```python
from build123d import *

# Parameters (mm, degrees)
SKETCH1_W           = 650
SKETCH1_H           = 250
SKETCH1_R           = 12.5
BOSS_EXTRUDE1_DEPTH = 119
SKETCH2_R           = 75
CUT_EXTRUDE1_DEPTH  = 267
FILLET1_R           = 50


with BuildPart() as part:
    # Sketch1 → Boss-Extrude1 (new body, symmetric)
    with BuildSketch(Plane(origin=(0, 0, 0), x_dir=(1, 0, 0), z_dir=(0, 1, 0))):
        Rectangle(SKETCH1_W, SKETCH1_H)
        with Locations((-250, -75)):
            Circle(SKETCH1_R, mode=Mode.SUBTRACT)
        with Locations((250, -75)):
            Circle(SKETCH1_R, mode=Mode.SUBTRACT)
        with Locations((250, 50)):
            Circle(SKETCH1_R, mode=Mode.SUBTRACT)
        with Locations((-250, 50)):
            Circle(SKETCH1_R, mode=Mode.SUBTRACT)
    extrude(amount=BOSS_EXTRUDE1_DEPTH, both=True)

    # Sketch2 → Cut-Extrude1 (cut)
    with BuildSketch(Plane.XY.offset(125)):
        with BuildLine():
            Line((-35.156791662, 87), (-325, 87))
            Line((-325, 87), (-325, -119))
            Line((-325, -119), (-5.04e-07, -119))
            ThreePointArc((-5.04e-07, -119), (-104.489233938, -30.832554252), (-35.156791662, 87))
        make_face()
        with BuildLine():
            Line((325, -119), (325, 87))
            Line((325, 87), (35.156791662, 87))
            ThreePointArc((35.156791662, 87), (104.489233853, -30.832554748), (-5.04e-07, -119))
            Line((-5.04e-07, -119), (325, -119))
        make_face()
        with Locations((0, -13)):
            Circle(SKETCH2_R)
    extrude(amount=-CUT_EXTRUDE1_DEPTH, mode=Mode.SUBTRACT)

    # Fillet1
    fillet1_edges = [part.edges().sort_by_distance(p)[0] for p in [
        (-35.156791662, 87, 0),
        (35.156791662, 87, 0),
    ]]
    fillet(fillet1_edges, radius=FILLET1_R)


solid = part.part
```
For this review, take the finished solid that the model builds, in its own axes (mm). A direction names the side the tool comes from. Give positions to 0.01 mm unless a question says otherwise; leave off trailing zeros. Write each loop counter-clockwise with the first axis right and the second up, starting at its lowest first coordinate (ties: lowest second). Pieces come first, ordered by that corner, then holes.
Item 1: Take a section at B-B (y = -13). Give the boundary of the cut face in (x, z), and give its area (3 significant figures).
Item 2: Insertion check: P1, Ø5, axis at x = 55.5, z = -18.5, coming from the -Y side; P2, Ø2, axis at y = -35.5, z = -71, coming from the +X side; P3, Ø1, axis at x = 76.5, z = 5.5, coming from the -Y side. Each pin has a flat end and moves straight along its axis. Give the tip position at first contact, or say it passes through.
Item 3: Machinability: for faces 1 (the face through (261.923, 102.776, -53.755)), 2 (the face through (238, 87, 2)), which of the approach directions +Z, -Z, +X, -X, +Y, -Y give a long, thin tool a straight path to every point of the face, cutting with its end or side? Answer none if there is none.
Item 4: The part is to be moulded in two halves that separate along Y. For faces 3 (the face through (-235, 87, 2)), 4 (the face through (-5, 119, -2)), 5 (the face through (-325, 103, 2)), 6 (the face through (107.53, 66.68, -1.75)), say which applies: +Y half, -Y half, draft (parallel to the pull), parting line (faces both ways), or undercut.
Item 5: Take a section at A-A (x = -250). Give the boundary of the cut face in (y, z), and give its area (3 significant figures).
Item 6: Wall thickness on probe 1 along X at (y, z) = (96, 75); probe 2 along Z at (x, y) = (250, 107); probe 3 along Y at (x, z) = (0, -1): over which ranges is each line inside the solid? List them lowest first.
Item 7: Take a section at C-C (z = 75). Give the boundary of the cut face in (x, y).
Item 8: Take a section at D-D (x = -65). Give the boundary of the cut face in (y, z), and give its area (3 significant figures).
Established:
1. outline: (-106, -125) - (-75, -125) - (-75, 125) - (-106, 125) - close; (75, -125) - (106, -125) - (106, 125) - (75, 125) - close
1. area: 15,500 mm2
2. P1: stops at y = -104.8
2. P2: stops at x = 103.8
2. P3: stops at y = -86.89
3. face 1: +Y, -Y
3. face 2: +Z, -Z, +X, -Y
4. face 3: -Y half
4. face 4: +Y half
4. face 5: draft
4. face 6: undercut
5. outline: (87, -125) - (119, -125) - (119, -62.5) - (87, -62.5) - close; (87, -37.5) - (119, -37.5) - (119, 62.5) - (87, 62.5) - close; (87, 87.5) - (119, 87.5) - (119, 125) - (87, 125) - close
5. area: 6,400 mm2
6. probe 1: x = -325 to -262.5, -237.5 to 237.5, 262.5 to 325
6. probe 2: z = -125 to -62.5, -37.5 to 62.5, 87.5 to 125
6. probe 3: y = -119 to -88, 62 to 119
7. outline: (-325, 87) - (-262.5, 87) - (-262.5, 119) - (-325, 119) - close; (-237.5, 87) - (-147.77, 87) arc R50 cw to (-100.41, 20.97) arc R106 ccw (long way) to (100.41, 20.97) arc R50 cw to (147.77, 87) - (237.5, 87) - (237.5, 119) - (-237.5, 119) - close; (262.5, 87) - (325, 87) - (325, 119) - (262.5, 119) - close; hole circle Ø150 at (0, -13)
8. outline: (-96.73, -125) - (-50.42, -125) - (-50.42, 125) - (-96.73, 125) - close; (24.42, -125) - (119, -125) - (119, 125) - (24.42, 125) - close
8. area: 35,200 mm2
